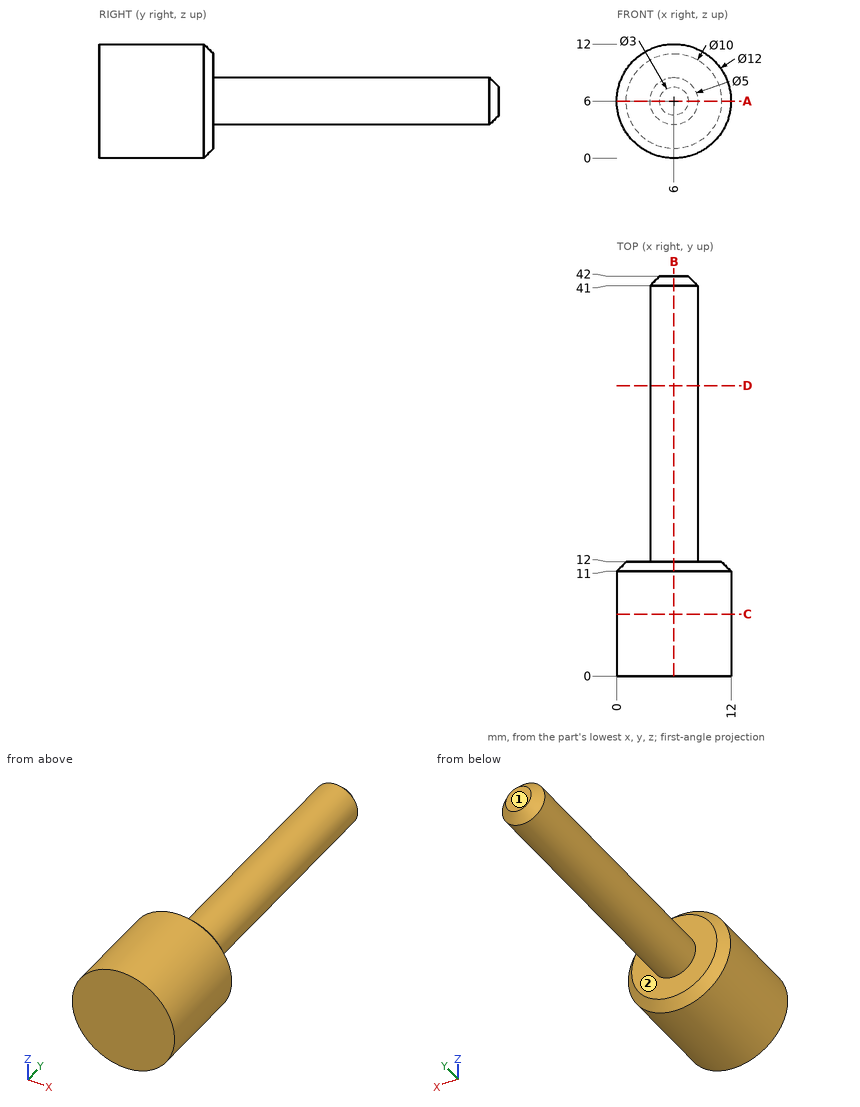
Job drawing, mm, ordinate dimensions from the low corner. One solid piece. A direction names the side the tool comes from. Round coordinates to 2 decimals unless told otherwise and drop trailing zeros. Loops run counter-clockwise (first coordinate to the right, second up) from the corner with the lowest first, then second, coordinate; pieces in that order, holes last.
(1) Cut at A-A (z = 6). Give the cut face in (x, y), plus the area to 3 significant figures.
(2) Wall check: line 1 along Y through (x, z) = (3.5, 8); line 2 along Z through (x, y) = (4, 28). Give the ranges that are in metal, low to high.
(3) Cut at D-D (y = 30.5). Give the cut face in (x, z).
(4) Cut at B-B (x = 6). Give the cut face in (y, z).
(5) Which spindle directions (+Z, -Z, +X, -X, +Y, -Y) get a long thin tool onto all of the face, cutting with end or side? Do the marked faces 1 and 2. Say none if no direction does.
(6) Drop flat-ended pins along their axis: pin 1 (2 mm diameter, centred on y = 20.5, z = 4, fed in from +X); pin 2 (4 mm diameter, centred on x = 9.5, z = 10.5, fed in from +Y). Give the stop position or say it passes through.
(7) Cut at C-C (y = 6.5). Give the cut face in (x, z).
Findings below:
1. outline: (0, 0) - (12, 0) - (12, 11) - (11, 12) - (8.5, 12) - (8.5, 41) - (7.5, 42) - (4.5, 42) - (3.5, 41) - (3.5, 12) - (1, 12) - (0, 11) - close
1. area: 292 mm2
2. line 1: y = 0 to 12
2. line 2: z = 4.5 to 7.5
3. outline: circle Ø5 at (6, 6)
4. outline: (0, 0) - (11, 0) - (12, 1) - (12, 3.5) - (41, 3.5) - (42, 4.5) - (42, 7.5) - (41, 8.5) - (12, 8.5) - (12, 11) - (11, 12) - (0, 12) - close
5. face 1: +Z, -Z, +X, -X, +Y
5. face 2: +Y
6. pin 1: stops at x = 8.29
6. pin 2: stops at y = 12
7. outline: circle Ø12 at (6, 6)
